Geometry: final body of the model. Coordinates: model frame, mm. A direction names the side the tool comes from. Give positions to 0.01 mm unless a question says otherwise; leave off trailing zeros. Write each loop counter-clockwise with the first axis right and the second up, starting at its lowest first coordinate (ties: lowest second). Pieces come first, ordered by that corner, then holes.
Q1. Line query: line 1 (Y direction, x = -68.5, z = -1.6); line 2 (X direction, y = -14, z = 1.4); line 3 (Y direction, x = -37, z = 0.15). Output: solid intervals per line, ascending.
Q2. Section C-C (y = -56). Return the cut outline in (x, z).
Q3. Section A-A (y = -116.5). Return the cut outline in (x, z), plus the area to 3 significant figures.
Q4. Section D-D (z = -0.5). State how many separate pieces and enclosed holes the cut face has, plus the area to 3 significant figures.
Q5. Reachability of faces 5 (the flat face through (-17.885, -55.981, 0.035)), 6 (the cylindrical face through (2.855, 4.73, 0.035)) from +Z, -Z, +X, -X, +Y, -Y: full face, straight path, thin tool, end or side. Return the list, or none.
Q6. Section B-B (x = -91.5). Return the cut outline in (y, z), plus the area to 3 significant figures.
Q7. Pin query (flat end, axial travel): pin 1 Ø2 at (x, z) = (-33, 0) entering from +Y; pin 2 Ø1.8 at (x, y) = (-85.22, -97.42) entering from +Z; pin 3 Ø1 at (y, z) = (-85, -1) entering from +X; pin 4 Ø1.5 at (x, z) = (-100.5, -1.5) entering from +Y. Return the tip coordinate at first contact, or that it passes through.
Q8. Mould query, pull axis X, two halves, no side actions, for faces 1 (the flat face through (-18.53, -26.164, 0.035)), 2 (the flat face through (-50.06, -21.16, 0.04)), 3 (the flat face through (-40, -68, -2.5)), 4 (the cylindrical face through (4.008, -130.727, 0.035)). Classes: +X half, -X half, draft (parallel to the pull), parting line (faces both ways), or undercut.
from build123d import *

# Parameters (mm, degrees)
SKETCH_1_R               = 18.5
SKETCH_1_R_2             = 1.525
SKETCH_1_R_3             = 3
EXTRUDE_1_DEPTH          = 2.5
SKETCH_4_R               = 1.525
CUT_EXTRUDE_3_DEPTH      = 10
PATTERN_CIRCULAR_2_COUNT = 6
SKETCH_5_R               = 1.525
CUT_EXTRUDE_4_DEPTH      = 31.54
CUT_EXTRUDE_5_DEPTH      = 31.54
EXTRUDE_2_DEPTH          = 5
EXTRUDE_3_DEPTH          = 5
FILLET_START             = -2.5
FILLET_2_DEPTH           = 5
CUT_EXTRUDE_7_DEPTH      = 5
FILLET_4_R               = 1.2


with BuildPart() as part:
    # 草图1 → 凸台-拉伸1 (new, symmetric)
    with BuildSketch(Plane.XY):
        with BuildLine():
            Line((-94.548784095, -99.337249729), (-2.310865067, -131.595640783))
            ThreePointArc((-2.310865067, -131.595640783), (4.084783214, -130.672665207), (6.99951255, -124.905468856))
            Line((6.99951255, -124.905468856), (5.524615263, 0.065201219))
            ThreePointArc((5.524615263, 0.065201219), (2.786503665, 4.770851321), (-2.657304464, 4.84400227))
            Line((-2.657304464, 4.84400227), (-98.809915302, -47.903033704))
            ThreePointArc((-98.809915302, -47.903033704), (-113.376342219, -75.003424702), (-94.548784095, -99.337249729))
        make_face()
        with Locations((-85.222792931, -72.671009109)):
            Circle(SKETCH_1_R, mode=Mode.SUBTRACT)
        Circle(SKETCH_1_R_2, mode=Mode.SUBTRACT)
        with Locations((0, -124.988076735)):
            Circle(SKETCH_1_R_3, mode=Mode.SUBTRACT)
    extrude(amount=EXTRUDE_1_DEPTH, both=True)

    # 草图4 → 切除-拉伸3 (cut)
    with BuildSketch(Plane.XY.offset(2.5)):
        with Locations((-85.222792931, -47.921009109)):
            Circle(SKETCH_4_R)
    cut_extrude_3 = extrude(amount=-CUT_EXTRUDE_3_DEPTH, mode=Mode.SUBTRACT)

    # 阵列(圆周)2: 切除-拉伸3 ×6 about axis
    pattern_circular_2_axis = Axis((-85.222792931, -72.671009109, 0), (0, 0, 1))
    for i in range(1, PATTERN_CIRCULAR_2_COUNT):
        add(cut_extrude_3.rotate(pattern_circular_2_axis, i * 360 / PATTERN_CIRCULAR_2_COUNT), mode=Mode.SUBTRACT)

    # 草图5 → 切除-拉伸4 (cut)
    with BuildSketch(Plane.XY.offset(2.5)):
        with Locations((-0.655427857, -29.992839384)):
            Circle(SKETCH_5_R)
        with Locations((-26.302274767, -14.428802517)):
            Circle(SKETCH_5_R)
    extrude(amount=-CUT_EXTRUDE_4_DEPTH, mode=Mode.SUBTRACT)

    # 草图6 → 切除-拉伸5 (cut)
    with BuildSketch(Plane.XY.offset(2.5)):
        with BuildLine():
            Line((-75.094363285, -46.299103359), (-27.959039434, -20.441785485))
            Line((-27.959039434, -20.441785485), (-4.062911687, -34.943381511))
            Line((-4.062911687, -34.943381511), (-3.124682468, -114.441211823))
            ThreePointArc((-3.124682468, -114.441211823), (-6.418945051, -116.055151994), (-8.999327109, -118.662563983))
            Line((-8.999327109, -118.662563983), (-70.892608691, -97.016610758))
            ThreePointArc((-70.892608691, -97.016610758), (-57.069243644, -70.338593517), (-75.094363285, -46.299103359))
        make_face()
    extrude(amount=-CUT_EXTRUDE_5_DEPTH, mode=Mode.SUBTRACT)

    # 草图7 → 凸台-拉伸2 (add)
    with BuildSketch(Plane.XY.offset(2.5)):
        with BuildLine():
            Line((-65.109328248, -99.039198909), (-60.447667843, -100.669522597))
            Line((-60.447667843, -100.669522597), (-3.986848357, -41.388362786))
            Line((-3.986848357, -41.388362786), (-4.062911687, -34.943381511))
            Line((-4.062911687, -34.943381511), (-8.001104314, -32.553451262))
            Line((-8.001104314, -32.553451262), (-64.766339632, -92.154233135))
            ThreePointArc((-64.766339632, -92.154233135), (-67.660383733, -94.798464524), (-70.892608691, -97.016610758))
            Line((-70.892608691, -97.016610758), (-65.109328248, -99.039198909))
        make_face()
    extrude(amount=-EXTRUDE_2_DEPTH)

    # 草图8 → 凸台-拉伸3 (add)
    with BuildSketch(Plane(origin=(0, 0, -2.5), x_dir=(-1, 0, 0), z_dir=(0, 0, -1))):
        Polygon((8.398824834, -119.639882413), (35.254100893, -72.768938625), (29.6986281, -68.384501663), (2.325139246, -116.159890547), align=None)
    extrude(amount=-EXTRUDE_3_DEPTH)

    # 圆角2: read off the stored shape, not the designer's step
    # 圆角2 outline → 圆角2 (add)
    with BuildSketch(Plane.XY.offset(FILLET_START)):
        with BuildLine():
            ThreePointArc((-52.068137932, -78.821728734), (-55.534618391, -79.459237326), (-57.214804329, -76.360870144))
            ThreePointArc((-57.214804329, -76.360870144), (-59.736362996, -84.857246804), (-64.766339632, -92.154233135))
            Line((-64.766339632, -92.154233135), (-52.068137932, -78.821728734))
        make_face()
        with BuildLine():
            ThreePointArc((-75.094363285, -46.299103359), (-73.733280759, -46.862994656), (-72.403446669, -47.497076929))
            ThreePointArc((-72.403446669, -47.497076929), (-73.222596192, -46.183465315), (-72.444213542, -44.845294226))
            Line((-72.444213542, -44.845294226), (-75.094363285, -46.299103359))
        make_face()
        with BuildLine():
            ThreePointArc((-9.594656237, -31.586388879), (-8.885938003, -32.671073224), (-9.286674719, -33.903238695))
            Line((-9.286674719, -33.903238695), (-8.001104314, -32.553451262))
            Line((-8.001104314, -32.553451262), (-9.594656237, -31.586388879))
        make_face()
        with BuildLine():
            Line((-27.959039434, -20.441785485), (-28.718320704, -20.858309136))
            ThreePointArc((-28.718320704, -20.858309136), (-27.964109185, -20.673780905), (-27.218678735, -20.891080529))
            Line((-27.218678735, -20.891080529), (-27.959039434, -20.441785485))
        make_face()
        with BuildLine():
            ThreePointArc((-6.52942074, -44.057942172), (-4.894363129, -43.696477917), (-3.943341833, -45.074747954))
            Line((-3.943341833, -45.074747954), (-3.986848357, -41.388362786))
            Line((-3.986848357, -41.388362786), (-6.52942074, -44.057942172))
        make_face()
        with BuildLine():
            ThreePointArc((-3.282371439, -114.489217858), (-3.203616876, -114.464919466), (-3.124682468, -114.441211823))
            ThreePointArc((-3.124682468, -114.441211823), (-3.391983975, -114.215991533), (-3.599904234, -113.93502278))
            Line((-3.599904234, -113.93502278), (-3.282371439, -114.489217858))
        make_face()
        with BuildLine():
            ThreePointArc((-29.142637234, -69.354881433), (-29.330280124, -68.429053989), (-28.927316541, -67.57466142))
            Line((-28.927316541, -67.57466142), (-29.6986281, -68.384501663))
            Line((-29.6986281, -68.384501663), (-29.142637234, -69.354881433))
        make_face()
        with BuildLine():
            ThreePointArc((-36.123402256, -75.130207215), (-34.857103993, -74.675567741), (-33.73571484, -75.419002143))
            Line((-33.73571484, -75.419002143), (-34.7358881, -73.67338372))
            Line((-34.7358881, -73.67338372), (-36.123402256, -75.130207215))
        make_face()
        with BuildLine():
            Line((-8.976957664, -118.630857917), (-9.129347243, -118.364889943))
            ThreePointArc((-9.129347243, -118.364889943), (-9.05625561, -118.510197041), (-8.999327109, -118.662563983))
            ThreePointArc((-8.999327109, -118.662563983), (-8.988156367, -118.646701086), (-8.976957664, -118.630857917))
        make_face()
        with BuildLine():
            ThreePointArc((-58.2536461, -101.436838383), (-59.216649338, -100.372621972), (-58.844644089, -98.986424331))
            Line((-58.844644089, -98.986424331), (-60.447667843, -100.669522597))
            Line((-60.447667843, -100.669522597), (-58.2536461, -101.436838383))
        make_face()
    extrude(amount=FILLET_2_DEPTH)

    # 草图12 → 切除-拉伸7 (cut)
    with BuildSketch(Plane.XY.offset(2.5)):
        Polygon((-3.112807373, -5.129369382), (-20.30370689, -14.559888089), (-3.541188361, -24.732384431), align=None)
    extrude(amount=-CUT_EXTRUDE_7_DEPTH, mode=Mode.SUBTRACT)

    # 圆角4
    fillet_4_edges = [part.edges().sort_by_distance(p)[0] for p in [
        (-3.112807373, -5.129369382, 0),
        (-3.541188361, -24.732384431, 0),
        (-20.30370689, -14.559888089, 0),
    ]]
    fillet(fillet_4_edges, radius=FILLET_4_R)


solid = part.part
Computed:
1. line 1: y = -108.45 to -80.58, -64.76 to -49.9, -42.68 to -31.28
1. line 2: x = -37.01 to -27.77, -24.84 to -18.94, -3.31 to 5.69
1. line 3: y = -119.46 to -108.87, -76.05 to -63, -25.4 to -14
2. outline: (-108.03, -2.5) - (-93.24, -2.5) - (-93.24, 2.5) - (-108.03, 2.5) - close; (-77.2, -2.5) - (-62.42, -2.5) - (-62.42, 2.5) - (-77.2, 2.5) - close; (-30.33, -2.5) - (-17.9, -2.5) - (-17.9, 2.5) - (-30.33, 2.5) - close; (-3.81, -2.5) - (6.19, -2.5) - (6.19, 2.5) - (-3.81, 2.5) - close
3. outline: (-45.47, -2.5) - (-15.18, -2.5) - (-15.18, 2.5) - (-45.47, 2.5) - close; (-10.2, -2.5) - (6.9, -2.5) - (6.9, 2.5) - (-10.2, 2.5) - close
3. area: 237 mm2
4. separate pieces: 1
4. enclosed holes: 15
4. area: 5,760 mm2
5. face 5: +Z, -Z
5. face 6: +Z, -Z, +Y
6. outline: (-100.4, -2.5) - (-90.07, -2.5) - (-90.07, 2.5) - (-100.4, 2.5) - close; (-55.27, -2.5) - (-43.89, -2.5) - (-43.89, 2.5) - (-55.27, 2.5) - close
6. area: 109 mm2
7. pin 1: stops at y = -11.25
7. pin 2: passes through
7. pin 3: stops at x = 6.53
7. pin 4: stops at y = -48.44
8. face 1: undercut
8. face 2: -X half
8. face 3: draft
8. face 4: parting line
